from build123d import *

# Parameters (mm, degrees)
F1_DEPTH = 2.5


with BuildPart() as f1:
    # F0 (on Front) → F1 (new body, symmetric)
    with BuildSketch(Plane.XZ):
        with BuildLine():
            Line((15.998854, 12.123694), (11.489416, 19.924695))
            Line((11.489416, 19.924695), (2.5, 19.919918))
            Line((2.5, 19.919918), (2.5, 32.854192))
            ThreePointArc((2.5, 32.854192), (0, 50.5), (-2.5, 32.854192))
            Line((-2.5, 32.854192), (-2.5, 19.917261))
            Line((-2.5, 19.917261), (-11.510584, 19.912474))
            Line((-11.510584, 19.912474), (-16.001155, 12.125023))
            Line((-16.001155, 12.125023), (-27.202565, 18.592159))
            ThreePointArc((-27.202565, 18.592159), (-43.734283, 25.25), (-29.702565, 14.262032))
            Line((-29.702565, 14.262032), (-18.498854, 7.793567))
            Line((-18.498854, 7.793567), (-23, -0.012222))
            Line((-23, -0.012222), (-18.501155, -7.794896))
            Line((-18.501155, -7.794896), (-29.702565, -14.262032))
            ThreePointArc((-29.702565, -14.262032), (-43.734283, -25.25), (-27.202565, -18.592159))
            Line((-27.202565, -18.592159), (-15.998854, -12.123694))
            Line((-15.998854, -12.123694), (-11.489416, -19.924695))
            Line((-11.489416, -19.924695), (-2.5, -19.919918))
            Line((-2.5, -19.919918), (-2.5, -32.854192))
            ThreePointArc((-2.5, -32.854192), (0, -50.5), (2.5, -32.854192))
            Line((2.5, -32.854192), (2.5, -19.917261))
            Line((2.5, -19.917261), (11.510584, -19.912474))
            Line((11.510584, -19.912474), (16.001155, -12.125023))
            Line((16.001155, -12.125023), (27.202565, -18.592159))
            ThreePointArc((27.202565, -18.592159), (43.734283, -25.25), (29.702565, -14.262032))
            Line((29.702565, -14.262032), (18.498854, -7.793567))
            Line((18.498854, -7.793567), (23, 0.012222))
            Line((23, 0.012222), (18.501155, 7.794896))
            Line((18.501155, 7.794896), (29.702565, 14.262032))
            ThreePointArc((29.702565, 14.262032), (43.734283, 25.25), (27.202565, 18.592159))
            Line((27.202565, 18.592159), (15.998854, 12.123694))
        make_face()
    extrude(amount=F1_DEPTH, both=True)


solid = f1.part
The listing builds one solid part. Answer for the finished solid, in the listing's coordinates (mm). A direction names the side the tool comes from. Coordinates: 2 decimals unless noted, no trailing zeros. Loops run counter-clockwise (first coordinate to the right, second up) from the corner with the lowest first, then second, coordinate; pieces in that order, holes last. Notation, with made-up numbers: (-23, -36.5) -> (-19, -36.5) arc R19 ccw to (-19, 0.5) -> close; hole circle Ø1 at (-36, -2). An arc over 180 degrees is marked (long way). Answer in a Markdown table with one row per item. Add a question column.
1. Consider line 1 (X direction, y = -0.4, z = -18.5); line 2 (Z direction, x = 22.5, y = 0.1); line 3 (X direction, y = 0, z = 23). Determine where each line is inside the solid, lowest interval first. Write a range as [from, to].
2. The part is cut by section C-C, the plane z = 21.5. Write down the section's boundary in (x, y), then the cut area to 3 significant figures.
3. Flat-ended cylindrical pins translate along their axes: P1, Ø3, axis at y = 0, z = 12, coming from the +X side; P2, Ø3, axis at x = -18.5, y = 0, coming from the +Z side; P3, Ø2, axis at y = 0.5, z = -40.5, coming from the +X side. Find the tip coordinate at first contact, or state that the pin passes through.
4. For faces 1 (the flat face through (24.02, -0.04, 10.98)), 2 (the flat face through (-13.776, -0.035, -15.97)), 3 (the flat face through (-20.718, -0.035, 3.945)), 4 (the flat face through (13.776, -0.035, 15.97)), determine the directions among +Z, -Z, +X, -X, +Y, -Y from which every point of the face is accessible in a straight line to the end or side of a thin tool.
5. The part is cut by section D-D, the plane z = -39. Write down the section's boundary in (x, y).
6. Determine the mould class of faces 5 (the flat face through (3, 2.5, 0)), 6 (the flat face through (-20.78, -0.04, -3.85)), 7 (the flat face through (2.5, 0, 26)) for opening direction X: +X half, -X half, draft (parallel to the pull), parting line (faces both ways), or undercut.
7. The part is cut by section A-A, the plane x = -4. Write down the section's boundary in (y, z), then the cut area to 3 significant figures.
Answer below:
| question | item | result |
|---|---|---|
| 1 | line 1 | [-44.65, -27.04], [-12.31, 12.33], [27.04, 44.65] |
| 1 | line 2 | [-15.88, -10.1], [-0.85, 0.88], [10.1, 15.88] |
| 1 | line 3 | [-44.65, -27.23], [-2.5, 2.5], [27.23, 44.65] |
| 2 | outline | (-44.91, -2.5) -> (-26.97, -2.5) -> (-26.97, 2.5) -> (-44.91, 2.5) -> close; (-2.5, -2.5) -> (2.5, -2.5) -> (2.5, 2.5) -> (-2.5, 2.5) -> close; (26.97, -2.5) -> (44.91, -2.5) -> (44.91, 2.5) -> (26.97, 2.5) -> close |
| 2 | area | 204 mm2 |
| 3 | P1 | x = 41.27 |
| 3 | P2 | z = 14.43 |
| 3 | P3 | x = 9 |
| 4 | face 1 | +Y, -Y |
| 4 | face 2 | -Z, +Y, -Y |
| 4 | face 3 | -X, +Y, -Y |
| 4 | face 4 | +Z, +Y, -Y |
| 5 | outline | (-8.65, -2.5) -> (8.65, -2.5) -> (8.65, 2.5) -> (-8.65, 2.5) -> close |
| 6 | face 5 | draft |
| 6 | face 6 | -X half |
| 6 | face 7 | undercut |
| 7 | outline | (-2.5, -49.56) -> (2.5, -49.56) -> (2.5, -33.44) -> (-2.5, -33.44) -> close; (-2.5, -19.92) -> (2.5, -19.92) -> (2.5, 19.92) -> (-2.5, 19.92) -> close; (-2.5, 33.44) -> (2.5, 33.44) -> (2.5, 49.56) -> (-2.5, 49.56) -> close |
| 7 | area | 360 mm2 |
